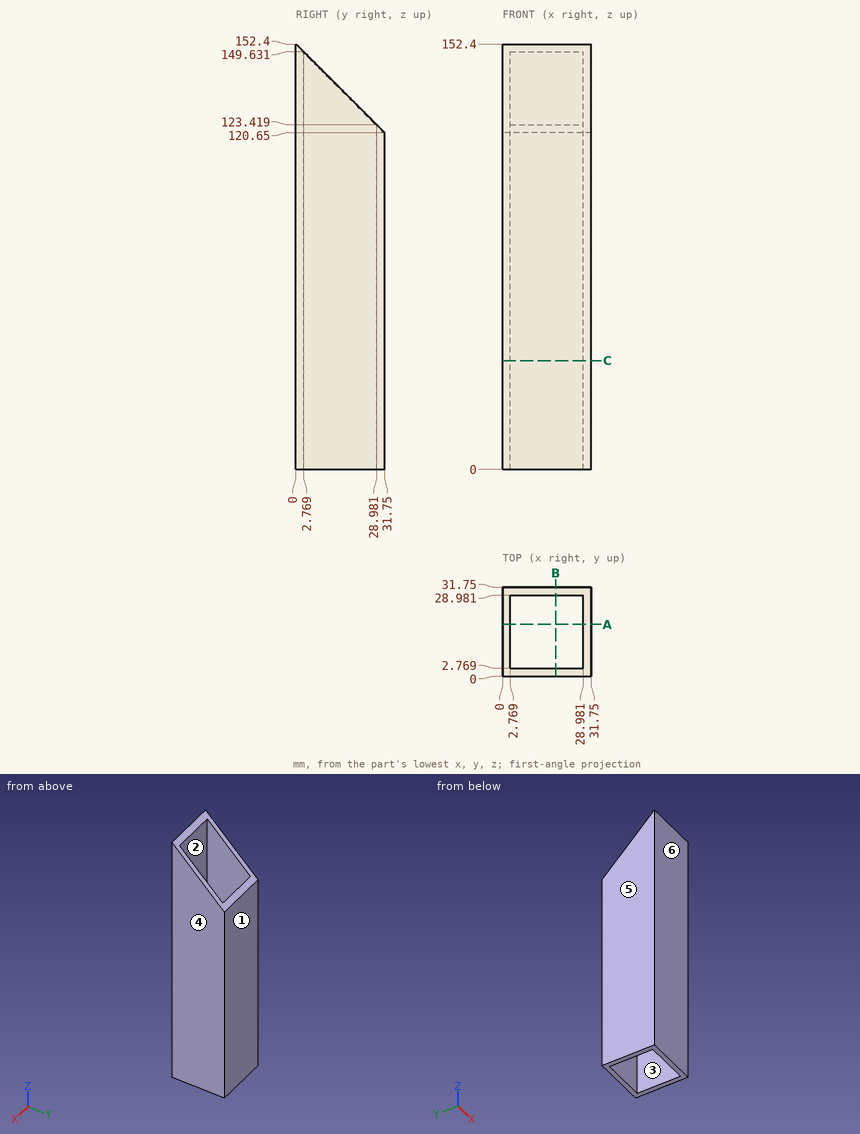
Check sheet for the drawn part. Datum: minimum x, y, z corner. Units: mm. A direction names the side the tool comes from. Round coordinates to 2 decimals unless told otherwise and drop trailing zeros. Order: outer loops, then holes, each group sorted by start corner. A loop starts at its lowest first (then second) coordinate and runs counter-clockwise, first axis right, second up.
1) Scan lines: line 1 (X direction, y = 13, z = 26); line 2 (Y direction, x = 18, z = 124.5). Record each from-to range of solid material in increasing order.
2) Tool access check on the marked faces 1 and 2. Record the directions out of +Z, -Z, +X, -X, +Y, -Y that give a thin tool (end or side, any length) a straight path to the whole face; none if there is none.
3) Mould release check, pull along X, two halves, no side actions. Record for the marked faces 3, 4, 5 and 6: +X half, -X half, draft (parallel to the pull), parting line (faces both ways), or undercut.
4) Section check C-C (z = 39). Record the boundary of the cut face in (x, y).
5) Section check A-A (y = 18.5). Record the boundary of the cut face in (x, z).
6) Section check B-B (x = 19). Record the boundary of the cut face in (y, z).
Result:
1. line 1: x = 0 to 2.77, 28.98 to 31.75
1. line 2: y = 0 to 2.77
2. face 1: +Z, -Z, +X, -X, +Y
2. face 2: +Z, -Z
3. face 3: undercut
3. face 4: +X half
3. face 5: -X half
3. face 6: draft
4. outline: (0, 0) - (31.75, 0) - (31.75, 31.75) - (0, 31.75) - close; hole (2.77, 2.77) - (28.98, 2.77) - (28.98, 28.98) - (2.77, 28.98) - close
5. outline: (0, 0) - (2.77, 0) - (2.77, 133.9) - (0, 133.9) - close; (28.98, 0) - (31.75, 0) - (31.75, 133.9) - (28.98, 133.9) - close
6. outline: (0, 0) - (2.77, 0) - (2.77, 149.63) - (0, 152.4) - close; (28.98, 0) - (31.75, 0) - (31.75, 120.65) - (28.98, 123.42) - close
